Part model, mm, in its own coordinate system. A direction names the side the tool comes from. Give positions to 0.01 mm unless a question says otherwise; leave off trailing zeros. Write each loop counter-clockwise with the first axis right and the second up, starting at its lowest first coordinate (ties: lowest second). Pieces come first, ordered by that corner, then holes. Notation, with made-up numbers: (78.5, 51) - (93.5, 51) arc R19 ccw to (93.5, 87) - close; hole circle Ø9 at (-38, 68.25). An arc over 180 degrees is marked (long way). Answer in a Markdown table with one row per item. Add a question column.
1. Which spindle directions (+Z, -Z, +X, -X, +Y, -Y) get a long thin tool onto all of the face, cutting with end or side? Do faces 1 (the cylindrical face through (13.368, 19.599, -0.035)), 2 (the cylindrical face through (-14.416, -21.011, -0.035)), 3 (the cylindrical face through (0.86, -24.045, -0.035)), 4 (the cylindrical face through (24.92, -4.67, -0.04)), 5 (the cylindrical face through (21.72, 12.816, -0.035)). Say none if no direction does.
2. Pull direction Y, two halves, no side cores. Call faces 6 (the cylindrical face through (11.978, 22.103, -0.035)), 7 (the cylindrical face through (-20.345, 12.252, -0.035)), 8 (the cylindrical face through (15.362, -20.358, -0.035)): released by +Y, released by -Y, zero draft, split by the parting line, or undercut.
3. Drop flat-ended pins along their axis: pin 1 Ø2 at (y, z) = (-8, 0) entering from +X; pin 2 Ø2 at (y, z) = (7, 0.5) entering from -X. Give the stop position or say it passes through.
4. Band-saw the part on B-B on x = -7. Write the cut outline in (y, z), plus the area to 3 significant figures.
5. Probe line 1 along Y through (x, z) = (-13.5, 1.6); line 2 along X through (y, z) = (16.5, -0.45); line 3 along X through (y, z) = (-16.5, -1.95). List the from-to ranges inside material, lowest first.
6. Band-saw the part on A-A on x = 6. Write the cut outline in (y, z), plus the area to 3 significant figures.
```python
from build123d import *

# Parameters (mm, degrees)
SKETCH1_R           = 27.75
BOSS_EXTRUDE1_DEPTH = 2.5
CUT_EXTRUDE2_START  = -5
CUT_EXTRUDE2_DEPTH  = 45.561660734
CIRPATTERN7_START   = -2.5
CIRPATTERN7_DEPTH   = 5


# Read off the part's stored shape, not the designer's step: CirPattern7
with BuildPart() as part:
    # Sketch1 → Boss-Extrude1 (new, symmetric)
    with BuildSketch(Plane.XY):
        Circle(SKETCH1_R)
    extrude(amount=BOSS_EXTRUDE1_DEPTH, both=True)

    # Sketch2 → Cut-Extrude2 (cut)
    with BuildSketch(Plane.XY.offset(2.5).offset(CUT_EXTRUDE2_START)):
        with BuildLine():
            Line((-89.477738944, 138.434122816), (-6.339011816, 27.016280817))
            ThreePointArc((-6.339011816, 27.016280817), (-5.280523031, 25.210404562), (-4.64520927, 23.215921174))
            ThreePointArc((-4.64520927, 23.215921174), (-2.923319917, 23.494917872), (-1.18556258, 23.646382525))
            ThreePointArc((-1.18556258, 23.646382525), (-1.058374477, 25.735739063), (-0.474695323, 27.745939601))
            Line((-0.474695323, 27.745939601), (52.825792272, 156.14002625))
            Line((52.825792272, 156.14002625), (18.496309012, 432.048381388))
            Line((18.496309012, 432.048381388), (-123.807222203, 414.342477955))
            Line((-123.807222203, 414.342477955), (-89.477738944, 138.434122816))
        make_face()
    extrude(amount=CUT_EXTRUDE2_DEPTH, mode=Mode.SUBTRACT)

    # CirPattern7 outline → CirPattern7 (cut)
    with BuildSketch(Plane.XY.offset(CIRPATTERN7_START)):
        with BuildLine():
            ThreePointArc((3.090231156, 23.479240771), (3.387839331, 24.901248443), (3.899737771, 26.260894145))
            ThreePointArc((3.899737771, 26.260894145), (4.000041355, 24.811544071), (3.877171664, 23.363932423))
            ThreePointArc((3.877171664, 23.363932423), (5.587296935, 23.020110291), (7.267466816, 22.551312602))
            ThreePointArc((7.267466816, 22.551312602), (7.814201579, 23.897328035), (8.560647715, 25.143720674))
            ThreePointArc((8.560647715, 25.143720674), (8.40054793, 23.699752356), (8.021171765, 22.297343653))
            ThreePointArc((8.021171765, 22.297343653), (9.642422807, 21.653692226), (11.211884607, 20.892422392))
            ThreePointArc((11.211884607, 20.892422392), (11.990173454, 22.119183541), (12.947175892, 23.212263034))
            ThreePointArc((12.947175892, 23.212263034), (12.531818479, 21.820086801), (11.9081293, 20.507955613))
            ThreePointArc((11.9081293, 20.507955613), (13.388397772, 19.585162378), (14.796707697, 18.555888238))
            ThreePointArc((14.796707697, 18.555888238), (15.781535783, 19.623965991), (16.918335679, 20.528599863))
            ThreePointArc((16.918335679, 20.528599863), (16.261070565, 19.232961405), (15.413114258, 18.053280708))
            ThreePointArc((15.413114258, 18.053280708), (16.704823111, 16.881004998), (17.906716922, 15.616808269))
            ThreePointArc((17.906716922, 15.616808269), (19.066431063, 16.491873729), (20.346490732, 17.178986303))
            ThreePointArc((20.346490732, 17.178986303), (19.468442959, 16.021528506), (18.423473536, 15.012214208))
            ThreePointArc((18.423473536, 15.012214208), (19.485106186, 13.628133929), (20.441954027, 12.169646935))
            ThreePointArc((20.441954027, 12.169646935), (21.739280055, 12.823574777), (23.121457326, 13.271081689))
            ThreePointArc((23.121457326, 13.271081689), (22.050848071, 12.289006199), (20.842451711, 11.482498492))
            ThreePointArc((20.842451711, 11.482498492), (21.63988641, 9.931099123), (22.320934405, 8.325198837))
            ThreePointArc((22.320934405, 8.325198837), (23.714175195, 8.736971281), (25.154045753, 8.930489292))
            ThreePointArc((25.154045753, 8.930489292), (23.92528528, 8.155360823), (22.592300834, 7.577581529))
            ThreePointArc((22.592300834, 7.577581529), (23.099907376, 5.908726323), (23.48326608, 4.207027699))
            ThreePointArc((23.48326608, 4.207027699), (24.927641727, 4.363410042), (26.378926948, 4.296719323))
            ThreePointArc((26.378926948, 4.296719323), (25.031508628, 3.753451142), (23.616779314, 3.422970562))
            ThreePointArc((23.616779314, 3.422970562), (23.818242806, 1.690297897), (23.891590756, -0.052505069))
            ThreePointArc((23.891590756, -0.052505069), (25.340677838, -0.156539085), (26.756732221, -0.481295039))
            ThreePointArc((26.756732221, -0.481295039), (25.333963188, -0.775241846), (23.88295957, -0.847801793))
            ThreePointArc((23.88295957, -0.847801793), (23.771804811, -2.588602391), (23.532784543, -4.316494579))
            ThreePointArc((23.532784543, -4.316494579), (24.940008208, -4.677601215), (26.2753186, -5.249984481))
            ThreePointArc((26.2753186, -5.249984481), (24.822927822, -5.285162221), (23.38228635, -5.0974694))
            ThreePointArc((23.38228635, -5.0974694), (22.962085944, -6.790447167), (22.418379767, -8.4478927))
            ThreePointArc((22.418379767, -8.4478927), (23.738510689, -9.054465692), (24.950159115, -9.856079401))
            ThreePointArc((24.950159115, -9.856079401), (23.514827626, -9.631357433), (22.130851702, -9.189444445))
            ThreePointArc((22.130851702, -9.189444445), (21.415111237, -10.780185683), (20.584194314, -12.313912898))
            ThreePointArc((20.584194314, -12.313912898), (21.774802399, -13.14645649), (22.823845482, -14.151536117))
            ThreePointArc((22.823845482, -14.151536117), (21.451706017, -13.67413719), (20.168877767, -12.992207482))
            ThreePointArc((20.168877767, -12.992207482), (19.180601729, -14.429584459), (18.089180414, -15.790298101))
            ThreePointArc((18.089180414, -15.790298101), (19.111998539, -16.822053658), (19.964719171, -17.998295117))
            ThreePointArc((19.964719171, -17.998295117), (18.699873422, -17.283563225), (17.559424, -16.38353458))
            ThreePointArc((17.559424, -16.38353458), (16.330376395, -17.621348817), (15.013529867, -18.76531443))
            ThreePointArc((15.013529867, -18.76531443), (15.835683816, -19.963120479), (16.464674853, -21.272718402))
            ThreePointArc((16.464674853, -21.272718402), (15.347776003, -20.343625616), (14.386360394, -19.254425694))
            ThreePointArc((14.386360394, -19.254425694), (12.956043823, -20.252892823), (11.456096612, -21.143342411))
            ThreePointArc((11.456096612, -21.143342411), (12.05116168, -22.46870048), (12.436206834, -23.869563312))
            ThreePointArc((12.436206834, -23.869563312), (11.503152931, -22.755971439), (10.751671822, -21.512608022))
            ThreePointArc((10.751671822, -21.512608022), (9.166057836, -22.239636488), (7.531219481, -22.847950269))
            ThreePointArc((7.531219481, -22.847950269), (7.880069787, -24.258262259), (8.00879339, -25.705365116))
            ThreePointArc((8.00879339, -25.705365116), (7.289573554, -24.443065915), (6.772180166, -23.085501726))
            ThreePointArc((6.772180166, -23.085501726), (5.082231704, -23.517724236), (3.365047255, -23.824350504))
            ThreePointArc((3.365047255, -23.824350504), (3.456470463, -25.274287827), (3.324735232, -26.721119633))
            ThreePointArc((3.324735232, -26.721119633), (2.84246578, -25.350684439), (2.575789563, -23.922552708))
            ThreePointArc((2.575789563, -23.922552708), (0.835822959, -24.046077275), (-0.908515864, -24.041160809))
            ThreePointArc((-0.908515864, -24.041160809), (-1.077458171, -25.484121288), (-1.465418157, -26.884179678))
            ThreePointArc((-1.465418157, -26.884179678), (-1.695236688, -25.449655405), (-1.702624541, -23.996857461))
            ThreePointArc((-1.702624541, -23.996857461), (-3.436685329, -23.807713904), (-5.152114041, -23.491412724))
            ThreePointArc((-5.152114041, -23.491412724), (-5.575991918, -24.88101842), (-6.207707306, -26.189304365))
            ThreePointArc((-6.207707306, -26.189304365), (-6.177688358, -24.736797805), (-5.925550396, -23.30602777))
            ThreePointArc((-5.925550396, -23.30602777), (-7.597971228, -22.810295317), (-9.229354538, -22.192775603))
            ThreePointArc((-9.229354538, -22.192775603), (-9.894544201, -23.484363447), (-10.749711139, -24.658827561))
            ThreePointArc((-10.749711139, -24.658827561), (-10.460819547, -23.235023468), (-9.957259691, -21.872267467))
            ThreePointArc((-9.957259691, -21.872267467), (-11.514287585, -21.085879369), (-13.009191491, -20.186988713))
            ThreePointArc((-13.009191491, -20.186988713), (-13.894313197, -21.339046008), (-14.945445916, -22.341940047))
            ThreePointArc((-14.945445916, -22.341940047), (-14.406966893, -20.992600658), (-13.668169972, -19.741658791))
            ThreePointArc((-13.668169972, -19.741658791), (-15.059760769, -18.689890207), (-16.370137831, -17.538519694))
            ThreePointArc((-16.370137831, -17.538519694), (-17.44674304, -18.514018371), (-18.660057269, -19.313108496))
            ThreePointArc((-18.660057269, -19.313108496), (-17.889297974, -18.081602688), (-16.939009528, -16.982681256))
            ThreePointArc((-16.939009528, -16.982681256), (-18.120436356, -15.699336894), (-19.204169976, -14.33249252))
            ThreePointArc((-19.204169976, -14.33249252), (-20.437655711, -15.100079248), (-21.774154532, -15.669682045))
            ThreePointArc((-21.774154532, -15.669682045), (-20.795887804, -14.595591428), (-19.664650885, -13.68401067))
            ThreePointArc((-19.664650885, -13.68401067), (-20.597941714, -12.210338274), (-21.420199801, -10.671951541))
            ThreePointArc((-21.420199801, -10.671951541), (-22.770920816, -11.206955453), (-24.187648058, -11.528763419))
            ThreePointArc((-24.187648058, -11.528763419), (-23.033316193, -10.64661015), (-21.757489688, -9.95166902))
            ThreePointArc((-21.757489688, -9.95166902), (-22.412647782, -8.335033634), (-22.947002286, -6.674549558))
            ThreePointArc((-22.947002286, -6.674549558), (-24.371545295, -6.959775187), (-25.822966179, -7.023445149))
            ThreePointArc((-25.822966179, -7.023445149), (-24.529670354, -6.361582359), (-23.150260375, -5.905616839))
            ThreePointArc((-23.150260375, -5.905616839), (-23.506228415, -4.197978453), (-23.735504741, -2.468766359))
            ThreePointArc((-23.735504741, -2.468766359), (-25.188083761, -2.495046318), (-26.627548424, -2.298531872))
            ThreePointArc((-26.627548424, -2.298531872), (-25.23685623, -1.878232376), (-23.79819815, -1.675897571))
            ThreePointArc((-23.79819815, -1.675897571), (-23.843535029, 0.067858911), (-23.760364049, 1.810220724))
            ThreePointArc((-23.760364049, 1.810220724), (-25.194291994, 2.043731094), (-26.575534859, 2.494113813))
            ThreePointArc((-26.575534859, 2.494113813), (-25.132144288, 2.659341243), (-23.68047776, 2.601542124))
            ThreePointArc((-23.68047776, 2.601542124), (-23.413726315, 4.325370935), (-23.020781211, 6.024881525))
            ThreePointArc((-23.020781211, 6.024881525), (-24.389970458, 6.510677009), (-25.668597242, 7.200452329))
            ThreePointArc((-25.668597242, 7.200452329), (-24.218900054, 7.105297148), (-22.800882836, 6.789221817))
            ThreePointArc((-22.800882836, 6.789221817), (-22.230616676, 8.43771768), (-21.540527028, 10.039753379))
            ThreePointArc((-21.540527028, 10.039753379), (-22.800970707, 10.762220109), (-23.935885294, 11.669218084))
            ThreePointArc((-23.935885294, 11.669218084), (-22.52647595, 11.316738658), (-21.187684281, 10.752546037))
            ThreePointArc((-21.187684281, 10.752546037), (-20.332232231, 12.272724938), (-19.367178088, 13.725794999))
            ThreePointArc((-19.367178088, 13.725794999), (-20.478364503, 14.661712301), (-21.433089803, 15.75678127))
            ThreePointArc((-21.433089803, 15.75678127), (-20.109267878, 15.158306577), (-18.892731625, 14.36413028))
            ThreePointArc((-18.892731625, 14.36413028), (-17.779588617, 15.70713242), (-16.570587613, 16.964533976))
            ThreePointArc((-16.570587613, 16.964533976), (-17.496802318, 18.083820698), (-18.240652676, 19.331764243))
            ThreePointArc((-18.240652676, 19.331764243), (-17.044966897, 18.506529753), (-15.989786535, 17.50789526))
            ThreePointArc((-15.989786535, 17.50789526), (-14.654729902, 18.630555443), (-13.240640324, 19.651874574))
            ThreePointArc((-13.240640324, 19.651874574), (-13.952114016, 20.918555919), (-14.461181467, 22.279264108))
            ThreePointArc((-14.461181467, 22.279264108), (-13.432062159, 21.253793536), (-12.572152054, 20.082797781))
            ThreePointArc((-12.572152054, 20.082797781), (-11.058091614, 20.949032787), (-9.484363464, 21.701443455))
            ThreePointArc((-9.484363464, 21.701443455), (-9.958228794, 23.074807243), (-10.216151493, 24.504545795))
            ThreePointArc((-10.216151493, 24.504545795), (-9.386675397, 23.311798609), (-8.749673767, 22.00607836))
            ThreePointArc((-8.749673767, 22.00607836), (-7.105272668, 22.588046681), (-5.422486865, 23.047365789))
            ThreePointArc((-5.422486865, 23.047365789), (-5.643513409, 24.483270978), (-5.642001509, 25.936086919))
            ThreePointArc((-5.642001509, 25.936086919), (-5.972131243, 26.488040866), (-6.339011816, 27.016280817))
            ThreePointArc((-6.339011816, 27.016280817), (3.426332111, -27.537660545), (-0.474695323, 27.745939601))
            ThreePointArc((-0.474695323, 27.745939601), (-0.700942634, 27.143900603), (-0.885748459, 26.527876571))
            ThreePointArc((-0.885748459, 26.527876571), (-0.528265346, 25.119728046), (-0.39067943, 23.673440882))
            ThreePointArc((-0.39067943, 23.673440882), (1.353355237, 23.640498771), (3.090231156, 23.479240771))
        make_face()
    extrude(amount=CIRPATTERN7_DEPTH, mode=Mode.SUBTRACT)


solid = part.part
```
Values:
| question | item | result |
|---|---|---|
| 1 | face 1 | +Z, -Z |
| 1 | face 2 | +Z, -Z, -X |
| 1 | face 3 | +Z, -Z, -Y |
| 1 | face 4 | +Z, -Z, +X |
| 1 | face 5 | +Z, -Z, +Y |
| 2 | face 6 | released by +Y |
| 2 | face 7 | undercut |
| 2 | face 8 | released by -Y |
| 3 | pin 1 | stops at x = 23.64 |
| 3 | pin 2 | stops at x = -25.67 |
| 4 | outline | (-23, -2.5) - (22.62, -2.5) - (22.62, 2.5) - (-23, 2.5) - close |
| 4 | area | 228 mm² |
| 5 | line 1 | y = -20.87 to 19.48, 20.06 to 21.33 |
| 5 | line 2 | x = -17.04 to 17.09, 19.08 to 19.87 |
| 5 | line 3 | x = -17.4 to 17.45, 17.69 to 18.83 |
| 6 | outline | (-23.3, -2.5) - (22.92, -2.5) - (22.92, 2.5) - (-23.3, 2.5) - close |
| 6 | area | 231 mm² |
